Read the model definition and answer for the solid it produces. Units are mm, in the model's axes. Face numbers are marked on the shaded views. A direction names the side the tool comes from. Give positions to 0.01 mm unless a question says otherwise; leave off trailing zeros. Loops run counter-clockwise (first coordinate to the right, second up) from the corner with the lowest first, then second, coordinate; pieces in that order, holes last. Notation, with made-up numbers: (15, 71) -> (47, 71) arc R17 cw to (47, 76) -> close; hole circle Ø6 at (-4, 31). An arc over 180 degrees is marked (long way). Answer as CSV lines item,"result". Start each with the question number.
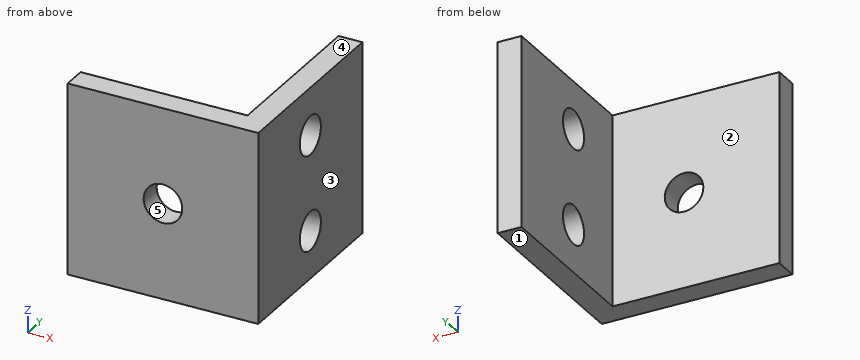
```python
from build123d import *

# Parameters (mm, degrees)
SKETCH_1_W          = 40
SKETCH_1_H          = 40
SKETCH_1_R          = 4.05
EXTRUDE_1_DEPTH     = 5
SKETCH_2_W          = 5
SKETCH_2_H          = 40
EXTRUDE_2_DEPTH     = 35
SKETCH_3_R          = 4.05
CUT_EXTRUDE_1_DEPTH = 35


with BuildPart() as part:
    # 草图1 → 凸台-拉伸1 (new body)
    with BuildSketch(Plane(origin=(0, 0, 0), x_dir=(1, 0, 0), z_dir=(0, 1, 0))):
        Rectangle(SKETCH_1_W, SKETCH_1_H)
        with Locations(Location((0, 0, 0), (0, 0, 270))):
            Circle(SKETCH_1_R, mode=Mode.SUBTRACT)
    extrude(amount=EXTRUDE_1_DEPTH)

    # 草图2 → 凸台-拉伸2 (add)
    with BuildSketch(Plane(origin=(0, 5, 0), x_dir=(1, 0, 0), z_dir=(0, 1, 0))):
        with Locations((17.5, 0)):
            Rectangle(SKETCH_2_W, SKETCH_2_H)
    extrude(amount=EXTRUDE_2_DEPTH)

    # 草图3 → 切除-拉伸1 (cut)
    with BuildSketch(Plane(origin=(20, 0, 0), x_dir=(0, 0, -1), z_dir=(1, 0, 0))):
        with Locations((-10, 20)):
            Circle(SKETCH_3_R)
        with Locations((10, 20)):
            Circle(SKETCH_3_R)
    extrude(amount=-CUT_EXTRUDE_1_DEPTH, mode=Mode.SUBTRACT)


solid = part.part
```
(1) Find section D-D on y = 3. Write down the section's boundary in (x, z).
(2) Each of these flat-tipped pins is pushed along its axis until it touches: P1, Ø5, axis at x = -14, z = 7, coming from the +Y side; P2, Ø10.5, axis at y = 16.5, z = 7.5, coming from the -X side; P3, Ø3, axis at x = -12.5, z = -5, coming from the -Y side; P4, Ø5, axis at y = 20, z = 10, coming from the +X side. Where does it stop, or does it pass through?
(3) Find section B-B on z = -10. Write down the section's boundary in (x, y), then the cut area to 4 significant figures.
(4) Find the intervals of material crossed by line 1 along X through (y, z) = (2.25, 0); line 2 along Y through (x, z) = (16, -10); line 3 along Y through (x, z) = (-2.5, -13), in increasing order. Write a range as from..to.
(5) Find section A-A on y = 20. Write down the section's boundary in (x, z).
(6) The mould has two halves that part along X. Classify the marked faces 3, 4 and 5: pulls with the +X half, pulls with the -X half, needs draft (parallel to the pull), parting line crosses it, or undercut.
(7) A tool of negligible diameter and unlimited length cuts with its end or side. For the marked faces 1 and 2, from which of +Z, -Z, +X, -X, +Y, -Y can it reach the whole face along a straight path? Write none if from no direction.
(8) Find section C-C on x = 0. Write down the section's boundary in (y, z).
Answer block:
1,outline,"(-20, -20) -> (20, -20) -> (20, 20) -> (-20, 20) -> close; hole circle Ø8.1 at (0, 0)"
2,P1,"stops at y = 5"
2,P2,"stops at x = 15"
2,P3,"stops at y = 0"
2,P4,"passes through"
3,outline,"(-20, 0) -> (20, 0) -> (20, 15.95) -> (15, 15.95) -> (15, 5) -> (-20, 5) -> close; (15, 24.05) -> (20, 24.05) -> (20, 40) -> (15, 40) -> close"
3,area,"334.5 mm2"
4,line 1,"x = -20..-4.05, 4.05..20"
4,line 2,"y = 0..15.95, 24.05..40"
4,line 3,"y = 0..5"
5,outline,"(15, -20) -> (20, -20) -> (20, -14.05) -> (15, -14.05) -> close; (15, -5.95) -> (20, -5.95) -> (20, 5.95) -> (15, 5.95) -> close; (15, 14.05) -> (20, 14.05) -> (20, 20) -> (15, 20) -> close"
6,face 3,"pulls with the +X half"
6,face 4,"needs draft"
6,face 5,"undercut"
7,face 1,"-Z, +X, -X, +Y, -Y"
7,face 2,"+Z, -Z, -X, +Y"
8,outline,"(0, -20) -> (5, -20) -> (5, -4.05) -> (0, -4.05) -> close; (0, 4.05) -> (5, 4.05) -> (5, 20) -> (0, 20) -> close"
